CAD build for the part. Positions are in the model's coordinates, mm. Give positions to 0.01 mm unless a question says otherwise; leave off trailing zeros. Loops run counter-clockwise (first coordinate to the right, second up) from the corner with the lowest first, then second, coordinate; pieces in that order, holes last.
```python
from build123d import *

# Parameters (mm, degrees)
SKETCH1_W           = 127
SKETCH1_H           = 127
BOSS_EXTRUDE1_DEPTH = 3.175
SKETCH2_R           = 3.25
CUT_EXTRUDE1_DEPTH  = 4.175


with BuildPart() as part:
    # Sketch1 → Boss-Extrude1 (new body)
    with BuildSketch(Plane(origin=(0, 0, 0), x_dir=(1, 0, 0), z_dir=(0, 1, 0))):
        with Locations((0, -25.4)):
            Rectangle(SKETCH1_W, SKETCH1_H)
    extrude(amount=BOSS_EXTRUDE1_DEPTH)

    # Sketch2 → Cut-Extrude1 (cut, through all)
    with BuildSketch(Plane(origin=(0, 3.175, 0), x_dir=(1, 0, 0), z_dir=(0, 1, 0))):
        Polygon((12.980662983, -43.432596685), (-63.5, 25.4), (-63.5, -88.9), (63.5, -88.9), (63.5, 12.7), align=None)
        with Locations((53, 28.1)):
            Circle(SKETCH2_R)
        with Locations((-53, 28.1)):
            Circle(SKETCH2_R)
    extrude(amount=-CUT_EXTRUDE1_DEPTH, mode=Mode.SUBTRACT)


solid = part.part
```
1. Saw through at A-A, the plane x = -53. List the corners of the cut face in (y, z) (3 decimals).
Responses:
outline: (0, -38.1) - (3.175, -38.1) - (3.175, -31.35) - (0, -31.35) - close; (0, -24.85) - (3.175, -24.85) - (3.175, -15.95) - (0, -15.95) - close
2. Saw through at D-D, the plane x = 53. List the corners of the cut face in (y, z) (3 decimals), and give its area (3 significant figures).
Responses:
outline: (0, -38.1) - (3.175, -38.1) - (3.175, -31.35) - (0, -31.35) - close; (0, -24.85) - (3.175, -24.85) - (3.175, -1.033) - (0, -1.033) - close
area: 97.0 mm2
3. Drop flat-ended pins along their axis: pin 1 (1 mm diameter, centred on y = 1, z = 21.5, fed in from -X); pin 2 (6 mm diameter, centred on x = -53, z = -28.1, fed in from +Y) (3 decimals). Give the stop position or say it passes through.
Responses:
pin 1: stops at x = -11.94
pin 2: passes through
4. Probe line 1 along X through (y, z) = (2.5, -28.1); line 2 along Z through (x, y) = (13, 2.45); line 3 along Z through (x, y) = (-53, 2.45). List the from-to ranges inside material, lowest first.
Responses:
line 1: x = -63.5 to -56.25, -49.75 to 49.75, 56.25 to 63.5
line 2: z = -38.1 to 43.41
line 3: z = -38.1 to -31.35, -24.85 to -15.95
5. Saw through at C-C, the plane y = 2.55. List the corners of the cut face in (x, z), and give its area (3 significant figures).
Responses:
outline: (-63.5, -38.1) - (63.5, -38.1) - (63.5, -12.7) - (12.98, 43.43) - (-63.5, -25.4) - close; hole circle Ø6.5 at (-53, -28.1); hole circle Ø6.5 at (53, -28.1)
area: 6,240 mm2
6. Pull direction Z, two halves, no side cores. Call faces 1 (the face through (54.75, 1.61, -30.84)), 2 (the face through (-1, 0, -7)), 3 (the face through (38.594, 1.61, 14.973)): released by +Z, released by -Z, zero draft, split by the parting line, or undercut.
Responses:
face 1: undercut
face 2: zero draft
face 3: released by +Z
7. Saw through at B-B, the plane z = -28.1. List the corners of the cut face in (x, y) (3 decimals).
Responses:
outline: (-63.5, 0) - (-56.25, 0) - (-56.25, 3.175) - (-63.5, 3.175) - close; (-49.75, 0) - (49.75, 0) - (49.75, 3.175) - (-49.75, 3.175) - close; (56.25, 0) - (63.5, 0) - (63.5, 3.175) - (56.25, 3.175) - close
